Source: CAD feature listing. Evaluate the final solid. Frame: model axes, mm. Face numbers are marked on the shaded views. A direction names the side the tool comes from. Coordinates: 2 decimals unless noted, no trailing zeros. Loops run counter-clockwise (first coordinate to the right, second up) from the corner with the lowest first, then second, coordinate; pieces in that order, holes last.
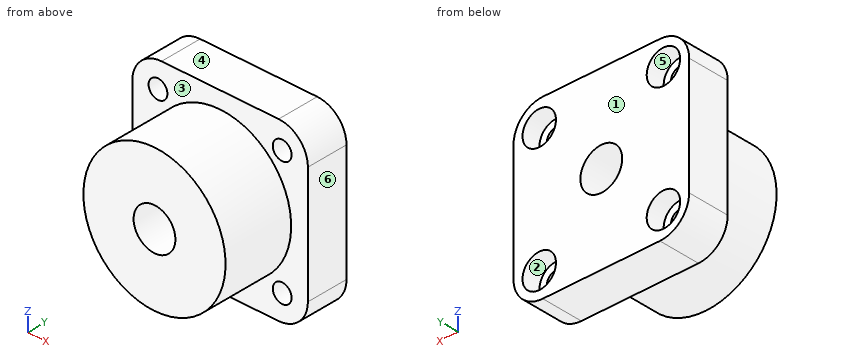
from build123d import *

# Parameters (mm, degrees)
SKETCH1_R                                           = 17
SKETCH1_R_2                                         = 5
BOSS_EXTRUDE1_DEPTH                                 = 17
SKETCH2_W                                           = 42
SKETCH2_H                                           = 42
SKETCH2_R                                           = 5
BOSS_EXTRUDE2_DEPTH                                 = 10
FILLET1_R                                           = 7
CBORE_FOR_M4_HEX_SOCKET_HEAD_CAP_SCREW1_D           = 4.5
CBORE_FOR_M4_HEX_SOCKET_HEAD_CAP_SCREW1_CBORE_D     = 8
CBORE_FOR_M4_HEX_SOCKET_HEAD_CAP_SCREW1_CBORE_DEPTH = 4.4


with BuildPart() as part:
    # Sketch1 → Boss-Extrude1 (new body)
    with BuildSketch(Plane(origin=(0, 0, 0), x_dir=(1, 0, 0), z_dir=(0, 1, 0))):
        with Locations(Location((0, 0, 0), (0, 0, 270))):
            Circle(SKETCH1_R)
        with Locations(Location((0, 0, 0), (0, 0, 270))):
            Circle(SKETCH1_R_2, mode=Mode.SUBTRACT)
    extrude(amount=BOSS_EXTRUDE1_DEPTH)

    # Sketch2 → Boss-Extrude2 (add)
    with BuildSketch(Plane(origin=(0, 17, 0), x_dir=(1, 0, 0), z_dir=(0, 1, 0))):
        Rectangle(SKETCH2_W, SKETCH2_H)
        with Locations(Location((0, 0, 0), (0, 0, 270))):
            Circle(SKETCH2_R, mode=Mode.SUBTRACT)
    extrude(amount=BOSS_EXTRUDE2_DEPTH)

    # Fillet1
    fillet1_edges = [part.edges().sort_by_distance(p)[0] for p in [
        (-21, 22, -21),
        (-21, 22, 21),
        (21, 22, 21),
        (21, 22, -21),
    ]]
    fillet(fillet1_edges, radius=FILLET1_R)

    # CBORE for M4 Hex Socket Head Cap Screw1 (through all)
    with Locations(Plane(origin=(-14.849242405, 27, -14.849242405), x_dir=(0, 0, 1), z_dir=(0, 1, 0))):
        with Locations((0, 0), (0, 29.69848481), (29.69848481, 29.69848481), (29.69848481, 0)):
            CounterBoreHole(CBORE_FOR_M4_HEX_SOCKET_HEAD_CAP_SCREW1_D / 2, CBORE_FOR_M4_HEX_SOCKET_HEAD_CAP_SCREW1_CBORE_D / 2, CBORE_FOR_M4_HEX_SOCKET_HEAD_CAP_SCREW1_CBORE_DEPTH)


solid = part.part
Q1. Contact query for flat-ended pins moving along their axis: pin 1 Ø2.5 at (x, z) = (-14, -13.5) entering from +Y; pin 2 Ø1 at (x, y) = (-6.5, 5.5) entering from -Z; pin 3 Ø3 at (y, z) = (12, 10.5) entering from -X; pin 4 Ø3.5 at (x, z) = (-14.85, 14.85) entering from +Y. Output: stop coordinate, or through.
Q2. Section B-B, the plane x = 0. Return the cut outline in (y, z), plus the area to 3 significant figures.
Q3. Section D-D, the plane z = 7.5. Return the cut outline in (x, y).
Q4. Section A-A, the plane z = 0. Return the cut outline in (x, y).
Q5. Draft query along X for the marked faces 4, 5 and 6. Return one class per face: +X half, -X half, draft (parallel to the pull), parting line (faces both ways), or undercut.
Q6. Section C-C, the plane y = 15. Return the cut outline in (x, z), plus the area to 3 significant figures.
Q7. Access query for the marked faces 1, 2 and 3. Directions: +Z, -Z, +X, -X, +Y, -Y. A direction counts if a zero-diameter tool reaches every point of the face in a straight line with its end or side. Return the directions, or none.
Q8. Line query: line 1 along Y through (x, z) = (13, 13.5); line 2 along X through (y, z) = (20.75, -4); line 3 along Y through (x, z) = (10, 15.5). Output: solid intervals per line, ascending.
Derived:
1. pin 1: stops at y = 22.6
1. pin 2: stops at z = -15.91
1. pin 3: stops at x = -14.42
1. pin 4: passes through
2. outline: (0, -17) - (17, -17) - (17, -21) - (27, -21) - (27, -5) - (0, -5) - close; (0, 5) - (27, 5) - (27, 21) - (17, 21) - (17, 17) - (0, 17) - close
2. area: 728 mm2
3. outline: (-21, 17) - (-15.26, 17) - (-15.26, 0) - (15.26, 0) - (15.26, 17) - (21, 17) - (21, 27) - (-21, 27) - close
4. outline: (-21, 17) - (-17, 17) - (-17, 0) - (-5, 0) - (-5, 27) - (-21, 27) - close; (5, 0) - (17, 0) - (17, 17) - (21, 17) - (21, 27) - (5, 27) - close
5. face 4: draft
5. face 5: undercut
5. face 6: +X half
6. outline: circle Ø34 at (0, 0); hole circle Ø10 at (0, 0)
6. area: 829 mm2
7. face 1: +Z, -Z, +X, -X, +Y
7. face 2: +Y
7. face 3: -Y
8. line 1: y = 17 to 22.6
8. line 2: x = -21 to -3, 3 to 21
8. line 3: y = 17 to 27
